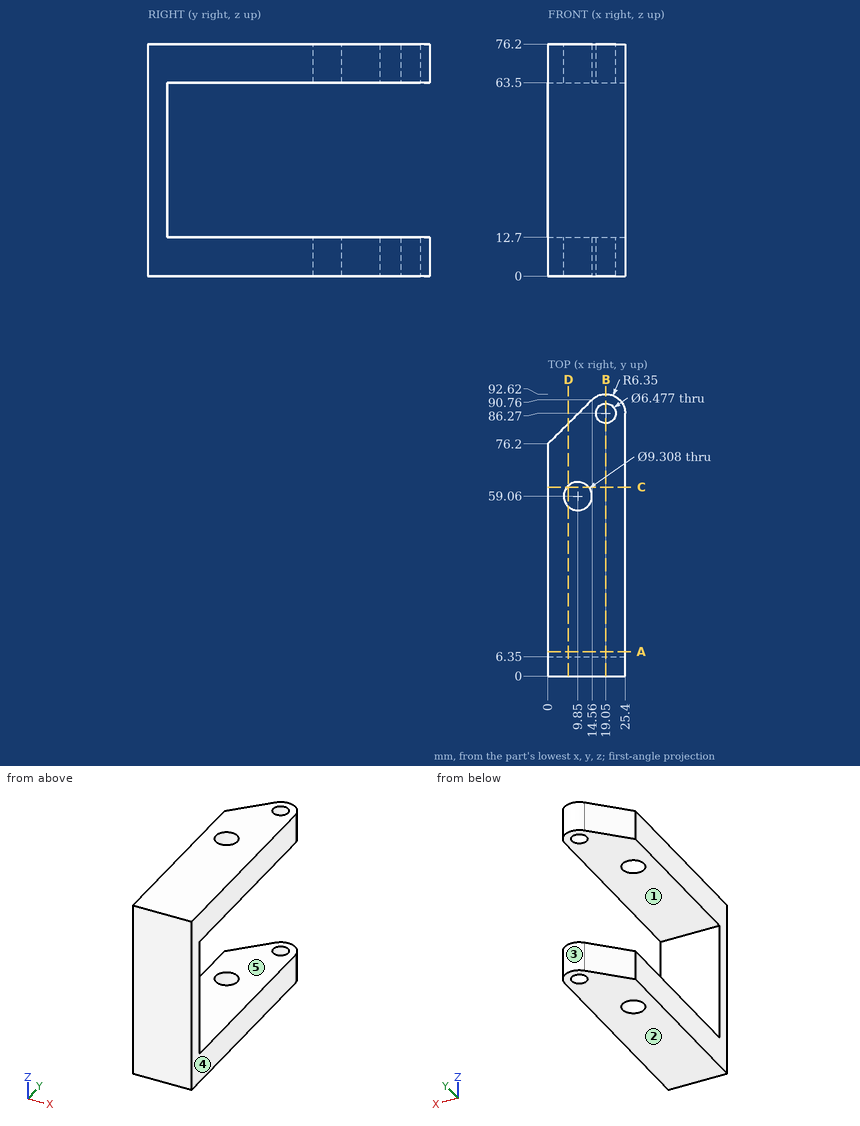
Input: dimensioned drawing with shaded views. Units: mm. Origin: part minimum x, y, z. A direction names the side the tool comes from. Coordinates: 2 decimals unless noted, no trailing zeros. Order: outer loops, then holes, each group sorted by start corner. A loop starts at its lowest first (then second) coordinate and runs counter-clockwise, first axis right, second up.
(1) Material intervals for probe 1 along Z at (x, y) = (14.75, 86); probe 2 along Y at (x, z) = (19.05, 71.5); probe 3 along Y at (x, z) = (20.25, 30.5), sorted ascending.
(2) First-contact query: pin 1 (6 mm diameter, centred on x = 19.5, y = 55.5, fed in from -Z); pin 2 (3 mm diameter, centred on x = 16.5, z = 8.5, fed in from +Y). Flat tips, straight axial feed; report the tip coordinate or a pass-through.
(3) Section query D-D (x = 6.75). Return the cut outline in (y, z), plus the area to 3 significant figures.
(4) Section query C-C (y = 62). Return the cut outline in (x, z).
(5) Section query A-A (y = 8). Return the cut outline in (x, z), plus the area to 3 significant figures.
(6) Access query for the marked faces 4 and 5. Directions: +Z, -Z, +X, -X, +Y, -Y. A direction counts if a zero-diameter tool reaches every point of the face in a straight line with its end or side. Return the directions, or none.
(7) Section query B-B (x = 19.05). Return the cut outline in (y, z).
(8) Draft query along Z for the marked faces 1, 2 and 3. Return one class per face: pulls with the +Z half, pulls with the -Z half, needs draft (parallel to the pull), parting line crosses it, or undercut.
Solution:
1. probe 1: z = 0 to 12.7, 63.5 to 76.2
1. probe 2: y = 0 to 83.03, 89.51 to 92.62
1. probe 3: y = 0 to 6.35
2. pin 1: stops at z = 0
2. pin 2: stops at y = 92.53
3. outline: (0, 0) - (55.59, 0) - (55.59, 12.7) - (6.35, 12.7) - (6.35, 63.5) - (55.59, 63.5) - (55.59, 76.2) - (0, 76.2) - close; (62.53, 0) - (82.95, 0) - (82.95, 12.7) - (62.53, 12.7) - close; (62.53, 63.5) - (82.95, 63.5) - (82.95, 76.2) - (62.53, 76.2) - close
3. area: 2,250 mm2
4. outline: (0, 0) - (6.24, 0) - (6.24, 12.7) - (0, 12.7) - close; (0, 63.5) - (6.24, 63.5) - (6.24, 76.2) - (0, 76.2) - close; (13.46, 0) - (25.4, 0) - (25.4, 12.7) - (13.46, 12.7) - close; (13.46, 63.5) - (25.4, 63.5) - (25.4, 76.2) - (13.46, 76.2) - close
5. outline: (0, 0) - (25.4, 0) - (25.4, 12.7) - (0, 12.7) - close; (0, 63.5) - (25.4, 63.5) - (25.4, 76.2) - (0, 76.2) - close
5. area: 645 mm2
6. face 4: +Z, -Z, +X, +Y, -Y
6. face 5: +X, -X, +Y
7. outline: (0, 0) - (83.03, 0) - (83.03, 12.7) - (6.35, 12.7) - (6.35, 63.5) - (83.03, 63.5) - (83.03, 76.2) - (0, 76.2) - close; (89.51, 0) - (92.62, 0) - (92.62, 12.7) - (89.51, 12.7) - close; (89.51, 63.5) - (92.62, 63.5) - (92.62, 76.2) - (89.51, 76.2) - close
8. face 1: undercut
8. face 2: pulls with the -Z half
8. face 3: needs draft
